Geometry: see drawing. Coordinates: mm, zero at the bounding-box minimum. Round coordinates to 2 decimals unless told otherwise and drop trailing zeros. Order: outer loops, then holes, each group sorted by start corner. A loop starts at its lowest first (then second) coordinate and runs counter-clockwise, first axis right, second up. Notation, with made-up numbers: (67.25, 86) -> (87.25, 86) arc R22 cw to (87.25, 112) -> close; hole circle Ø3 at (-18.5, -28.5). An arc over 180 degrees is marked (long way). Write item = value, one per line. Start each with the question number.
(1) Contact query for a flat-ended pin moving along its axis: pin 1 Ø7.5 at (x, y) = (7, 38) entering from +Z. Output: stop coordinate, or through.
(2) Ray query, line 1 (Y direction, x = 6.35, z = 26) (3 decimals); line 2 (X direction, y = 38, z = 73); line 3 (Y direction, x = 4, z = 5.5). Return the intervals inside material, ascending.
(3) Cut plane C-C on z = 58. Return the cut outline in (x, y) (3 decimals), then the cut area to 3 significant figures.
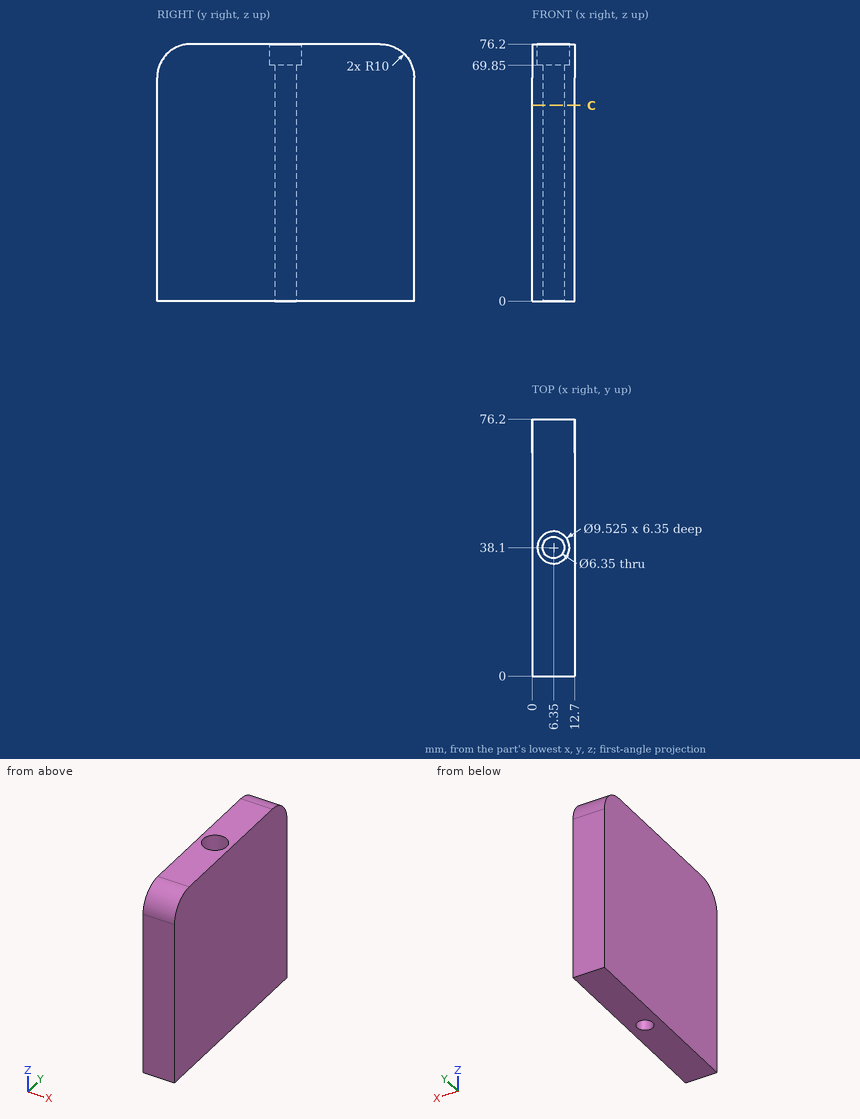
Evaluation:
q1.pin_1 = 69.85
q2.line_1 = 0 to 34.925, 41.275 to 76.2
q2.line_2 = 0 to 1.59, 11.11 to 12.7
q2.line_3 = 0 to 35.97, 40.23 to 76.2
q3.outline = (0, 0) -> (12.7, 0) -> (12.7, 76.2) -> (0, 76.2) -> close; hole circle Ø6.35 at (6.35, 38.1)
q3.area = 936 mm^2
